Source: CAD feature listing. Evaluate the final solid. Frame: model axes, mm. Face numbers are marked on the shaded views. A direction names the side the tool comes from. Round coordinates to 2 decimals unless told otherwise and drop trailing zeros. Loops run counter-clockwise (first coordinate to the right, second up) from the corner with the lowest first, then second, coordinate; pieces in that order, holes last. Notation, with made-up numbers: M 22,16 L 44,16 A21 ccw 44,39 Z; hole C -35.5,48 d3. An arc over 180 degrees is marked long. Answer as a JSON object with one key per item and string values.
from build123d import *

# Parameters (mm, degrees)
SKETCH_1_R          = 26.85
EXTRUDE_1_DEPTH     = 15
SKETCH_3_R          = 10
EXTRUDE_2_DEPTH     = 10
SKETCH_2_R          = 2.5
CUT_EXTRUDE_1_DEPTH = 46.462567019


with BuildPart() as part:
    # 스케치1 → 보스-돌출1 (new body)
    with BuildSketch(Plane(origin=(0, 0, 0), x_dir=(1, 0, 0), z_dir=(0, 1, 0))):
        with Locations(Location((0, 0, 0), (0, 0, 270))):
            Circle(SKETCH_1_R)
    extrude(amount=EXTRUDE_1_DEPTH)

    # 스케치3 → 보스-돌출2 (add)
    with BuildSketch(Plane(origin=(0, 15, 0), x_dir=(1, 0, 0), z_dir=(0, 1, 0))):
        with Locations(Location((0, 0, 0), (0, 0, 270))):
            Circle(SKETCH_3_R)
    extrude(amount=EXTRUDE_2_DEPTH)

    # 스케치2 → 컷-돌출1 (cut, through all)
    with BuildSketch(Plane.XZ):
        with Locations(Location((0, 0, 0), (0, 0, 270))):
            Circle(SKETCH_2_R)
    extrude(amount=-CUT_EXTRUDE_1_DEPTH, mode=Mode.SUBTRACT)


solid = part.part
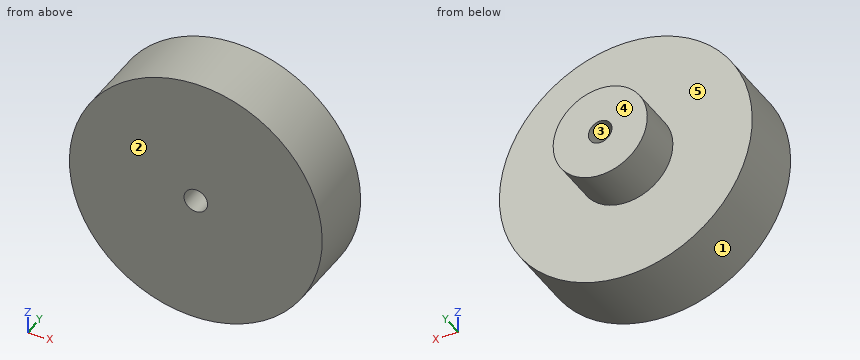
Item 1: Access query for the marked faces 4 and 5. Directions: +Z, -Z, +X, -X, +Y, -Y. A direction counts if a zero-diameter tool reaches every point of the face in a straight line with its end or side. Return the directions, or none.
Answer sheet:
{"face 4": "+Z, -Z, +X, -X, +Y", "face 5": "+Y"}
Item 2: Line query: probe 1 along X at (y, z) = (17, 0); probe 2 along X at (y, z) = (7.5, 0); probe 3 along Y at (x, z) = (-10, 10.5). Output: solid intervals per line, ascending. Write a range as from..to.
Answer sheet:
{"probe 1": "x = -10..-2.5, 2.5..10", "probe 2": "x = -26.85..-2.5, 2.5..26.85", "probe 3": "y = 0..15"}
Item 3: Pull-direction query (X, two-part tool) for the marked faces 1, 2 and 3; classes: pulls with the +X half, pulls with the -X half, needs draft (parallel to the pull), parting line crosses it, or undercut.
Answer sheet:
{"face 1": "parting line crosses it", "face 2": "needs draft", "face 3": "undercut"}
Item 4: Contact query for flat-ended pins moving along their axis: pin 1 Ø10 at (x, y) = (5, 11) entering from -Z; pin 2 Ø1 at (y, z) = (13, 21) entering from -X; pin 3 Ø2 at (y, z) = (8, 2) entering from -X; pin 4 Ø3 at (x, y) = (11, 12) entering from -Z. Output: stop coordinate, or through.
Answer sheet:
{"pin 1": "stops at z = -26.85", "pin 2": "stops at x = -17.34", "pin 3": "stops at x = -26.83", "pin 4": "stops at z = -25.11"}
Item 5: Section B-B on z = 0. Return the cut outline in (x, y), then the cut area to 4 significant figures.
Answer sheet:
{"outline": "M -26.85,0 L -2.5,0 L -2.5,25 L -10,25 L -10,15 L -26.85,15 Z; M 2.5,0 L 26.85,0 L 26.85,15 L 10,15 L 10,25 L 2.5,25 Z", "area": "880.5 mm²"}
Item 6: Section D-D on z = -8.5. Return the cut outline in (x, y), then the cut area to 3 significant figures.
Answer sheet:
{"outline": "M -25.47,0 L 25.47,0 L 25.47,15 L 5.27,15 L 5.27,25 L -5.27,25 L -5.27,15 L -25.47,15 Z", "area": "869 mm²"}
Item 7: Section C-C on y = 5. Return the cut outline in (x, z), then the cut area to 3 significant figures.
Answer sheet:
{"outline": "C 0,0 d53.7; hole C 0,0 d5", "area": "2,250 mm²"}
Item 8: Section A-A on x = 0. Return the cut outline in (y, z).
Answer sheet:
{"outline": "M 0,-26.85 L 15,-26.85 L 15,-10 L 25,-10 L 25,-2.5 L 0,-2.5 Z; M 0,2.5 L 25,2.5 L 25,10 L 15,10 L 15,26.85 L 0,26.85 Z"}
